from build123d import *

# Parameters (mm, degrees)
SKETCH_1_W             = 26
SKETCH_1_H             = 30
EXTRUDE_1_DEPTH        = 1.6
SKETCH_2_W             = 6
SKETCH_2_H             = 6
EXTRUDE_2_DEPTH        = 1
CUT_EXTRUDE_1_REACH    = 21.914
SKETCH_3_R             = 0.475
PATTERN_LINEAR_2_COUNT = 9
PATTERN_LINEAR_2_PITCH = 2.54


with BuildPart() as part:
    # Sketch 1 → Extrude 1 (new body)
    with BuildSketch(Plane.XY):
        Rectangle(SKETCH_1_W, SKETCH_1_H)
    extrude(amount=-EXTRUDE_1_DEPTH)

    # Sketch 2 → Extrude 2 (add)
    with BuildSketch(Plane.XY):
        with Locations((0, -2)):
            Rectangle(SKETCH_2_W, SKETCH_2_H)
    extrude(amount=EXTRUDE_2_DEPTH)

    # Sketch 3 → Cut-Extrude 1 (cut, up to next)
    with BuildSketch(Plane.XY, mode=Mode.PRIVATE) as cut_extrude_1_sk1:
        with Locations((-11.43, -13.73)):
            Circle(SKETCH_3_R)
    cut_extrude_1_tool1 = extrude(cut_extrude_1_sk1.sketch, amount=-CUT_EXTRUDE_1_REACH, mode=Mode.PRIVATE) & part.part
    # Sketch 3 → Cut-Extrude 1 (cut, up to next)
    with BuildSketch(Plane.XY, mode=Mode.PRIVATE) as cut_extrude_1_sk2:
        with Locations((11.43, -13.73)):
            Circle(SKETCH_3_R)
    cut_extrude_1_tool2 = extrude(cut_extrude_1_sk2.sketch, amount=-CUT_EXTRUDE_1_REACH, mode=Mode.PRIVATE) & part.part
    # Sketch 3 → Cut-Extrude 1 (cut, up to next)
    with BuildSketch(Plane.XY, mode=Mode.PRIVATE) as cut_extrude_1_sk3:
        with Locations((-8.89, -13.73)):
            Circle(SKETCH_3_R)
    cut_extrude_1_tool3 = extrude(cut_extrude_1_sk3.sketch, amount=-CUT_EXTRUDE_1_REACH, mode=Mode.PRIVATE) & part.part
    # Sketch 3 → Cut-Extrude 1 (cut, up to next)
    with BuildSketch(Plane.XY, mode=Mode.PRIVATE) as cut_extrude_1_sk4:
        with Locations((8.89, -13.73)):
            Circle(SKETCH_3_R)
    cut_extrude_1_tool4 = extrude(cut_extrude_1_sk4.sketch, amount=-CUT_EXTRUDE_1_REACH, mode=Mode.PRIVATE) & part.part
    cut_extrude_1_1 = cut_extrude_1_tool1.solids().sort_by_distance((-11.43, -13.73, 0))[0]
    add(cut_extrude_1_1, mode=Mode.SUBTRACT)
    cut_extrude_1_2 = cut_extrude_1_tool2.solids().sort_by_distance((11.43, -13.73, 0))[0]
    add(cut_extrude_1_2, mode=Mode.SUBTRACT)
    cut_extrude_1_3 = cut_extrude_1_tool3.solids().sort_by_distance((-8.89, -13.73, 0))[0]
    add(cut_extrude_1_3, mode=Mode.SUBTRACT)
    cut_extrude_1_4 = cut_extrude_1_tool4.solids().sort_by_distance((8.89, -13.73, 0))[0]
    add(cut_extrude_1_4, mode=Mode.SUBTRACT)
    cut_extrude_1 = cut_extrude_1_1 + cut_extrude_1_2 + cut_extrude_1_3 + cut_extrude_1_4  # Cut-Extrude 1 as one shape, for the pattern or mirror that repeats it

    # Pattern Linear 2: Cut-Extrude 1 ×9
    with Locations(*[(0, i * PATTERN_LINEAR_2_PITCH, 0) for i in range(1, PATTERN_LINEAR_2_COUNT)]):
        add(cut_extrude_1, mode=Mode.SUBTRACT)


solid = part.part
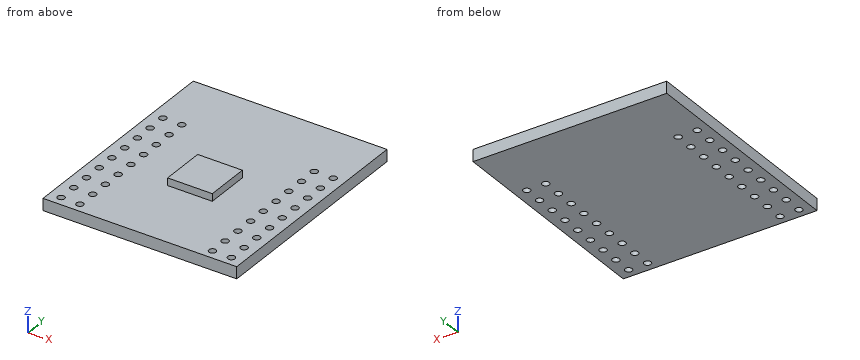
Input: part model. Units: mm. Frame: model coordinates. Coordinates: 2 decimals unless noted, no trailing zeros. Loops run counter-clockwise (first coordinate to the right, second up) from the corner with the lowest first, then second, coordinate; pieces in that order, holes last. Notation, with made-up numbers: (-34.75, -22.75) - (13.25, -22.75) arc R26 cw to (13.25, 5.25) - close; hole circle Ø2 at (-7.75, -15). An arc over 180 degrees is marked (long way). Answer in a Markdown table with one row per item. Add a question column.
Item 1: Section query C-C on z = -0.8. State how many separate pieces and enclosed holes the cut face has, then the cut area to 3 significant figures.
Item 2: Contact query for flat-ended pins moving along their axis: P1, Ø1.5, axis at x = 3, y = 8.5, coming from the +Z side; P2, Ø0.5, axis at x = -1.5, z = 0.5, coming from the -Y side; P3, Ø0.8, axis at x = -1.5, z = 0.5, coming from the +Y side. Output: stop coordinate, or through.
Item 3: Section query B-B on x = -2.25. Return the cut outline in (y, z).
Item 4: Section query A-A on y = -3.57. Return the cut outline in (x, z) (3 decimals).
Item 5: Section query D-D on y = -11.19. Return the cut outline in (x, z) (3 decimals).
Item 6: Line query: line 1 along X through (y, z) = (-11, -1.3); line 2 along Z through (x, y) = (-5.5, 6.5); line 3 along Y through (x, z) = (1.5, 0.6). Output: solid intervals per line, ascending. Write a range as [from, to].
Recorded:
| question | item | result |
|---|---|---|
| 1 | separate pieces | 1 |
| 1 | enclosed holes | 36 |
| 1 | area | 754 mm^2 |
| 2 | P1 | z = 0 |
| 2 | P2 | y = -5 |
| 2 | P3 | y = 1 |
| 3 | outline | (-15, -1.6) - (15, -1.6) - (15, 0) - (1, 0) - (1, 1) - (-5, 1) - (-5, 0) - (-15, 0) - close |
| 4 | outline | (-13, -1.6) - (-11.905, -1.6) - (-11.905, 0) - (-13, 0) - close; (-10.955, -1.6) - (-9.365, -1.6) - (-9.365, 0) - (-10.955, 0) - close; (-8.415, -1.6) - (8.415, -1.6) - (8.415, 0) - (3, 0) - (3, 1) - (-3, 1) - (-3, 0) - (-8.415, 0) - close; (9.365, -1.6) - (10.955, -1.6) - (10.955, 0) - (9.365, 0) - close; (11.905, -1.6) - (13, -1.6) - (13, 0) - (11.905, 0) - close |
| 5 | outline | (-13, -1.6) - (-11.905, -1.6) - (-11.905, 0) - (-13, 0) - close; (-10.955, -1.6) - (-9.365, -1.6) - (-9.365, 0) - (-10.955, 0) - close; (-8.415, -1.6) - (8.415, -1.6) - (8.415, 0) - (-8.415, 0) - close; (9.365, -1.6) - (10.955, -1.6) - (10.955, 0) - (9.365, 0) - close; (11.905, -1.6) - (13, -1.6) - (13, 0) - (11.905, 0) - close |
| 6 | line 1 | [-13, -11.87], [-10.99, -9.33], [-8.45, 8.45], [9.33, 10.99], [11.87, 13] |
| 6 | line 2 | [-1.6, 0] |
| 6 | line 3 | [-5, 1] |
